from build123d import *

# Parameters (mm, degrees)
SKETCH1_W                       = 15.875
SKETCH1_H                       = 34.925
BASE_FLANGE1_DEPTH              = 3.03784
F_9_32_0_28125_DIAMETER_HOLE1_D = 7.14375
BREAK_CORNER1_DEPTH             = 3.03784


# Read off the part's stored shape, not the designer's step: Break-Corner1
# Sheet-metal steps are written as plain solids
with BuildPart() as part:
    # Sketch1 → Base-Flange1 (new body)
    with BuildSketch(Plane.XY):
        Rectangle(SKETCH1_W, SKETCH1_H)
    extrude(amount=BASE_FLANGE1_DEPTH)

    # 9/32 (0.28125) Diameter Hole1 (through all)
    with Locations(Plane.XY.offset(3.03784)):
        with Locations((0, 9.525), (0, -9.525)):
            Hole(F_9_32_0_28125_DIAMETER_HOLE1_D / 2)

    # Break-Corner1 outline → Break-Corner1 (cut)
    with BuildSketch(Plane.XY):
        with BuildLine():
            Line((-7.9375, -17.4625), (-3.175, -17.4625))
            ThreePointArc((-3.175, -17.4625), (-6.542596045, -16.067596045), (-7.9375, -12.7))
            Line((-7.9375, -12.7), (-7.9375, -17.4625))
        make_face()
        with BuildLine():
            ThreePointArc((7.9375, -12.7), (6.542596045, -16.067596045), (3.175, -17.4625))
            Line((3.175, -17.4625), (7.9375, -17.4625))
            Line((7.9375, -17.4625), (7.9375, -12.7))
        make_face()
        with BuildLine():
            Line((-7.9375, 17.4625), (-7.9375, 12.7))
            ThreePointArc((-7.9375, 12.7), (-6.542596045, 16.067596045), (-3.175, 17.4625))
            Line((-3.175, 17.4625), (-7.9375, 17.4625))
        make_face()
        with BuildLine():
            ThreePointArc((3.175, 17.4625), (6.542596045, 16.067596045), (7.9375, 12.7))
            Line((7.9375, 12.7), (7.9375, 17.4625))
            Line((7.9375, 17.4625), (3.175, 17.4625))
        make_face()
    extrude(amount=BREAK_CORNER1_DEPTH, mode=Mode.SUBTRACT)


solid = part.part
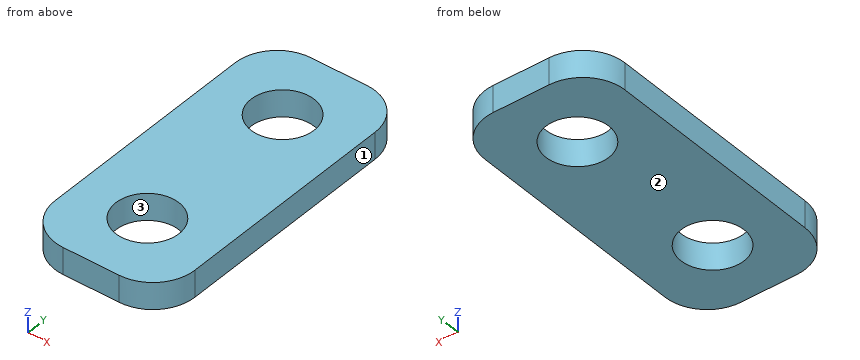
For this review, take the finished solid that the model builds, in its own axes (mm). Face numbers are marked on the shaded views. Give positions to 0.01 mm unless a question says otherwise; leave off trailing zeros. Loops run counter-clockwise (first coordinate to the right, second up) from the corner with the lowest first, then second, coordinate; pieces in that order, holes last. Notation, with made-up numbers: M 40,39 L 72,39 A12 cw 72,62 Z; hole C 17,-39 d6. An arc over 180 degrees is marked long. Put each result on its own line as item: value. Start each with the question number.
(1) Add section A-A, the plane x = 0. Write out the cut boundary in (y, z), then the cut area to 3 significant figures.
(2) Wall thickness on L1, parallel to Y at x = 0, z = 1.15; L2, parallel to Y at x = 3, z = 2; L3, parallel to X at y = -7, z = 2.35: over which ranges is each line inside the solid? List them lowest first.
(3) The part is to be moulded in two halves that separate along X. For the marked faces 1, 2 and 3, say which applies: +X half, -X half, draft (parallel to the pull), parting line (faces both ways), or undercut.
(4) For pin 1 (1 mm diameter, centred on x = -6, z = 2.5, fed in from -Y), flat-tipped, find the tip position at first contact; note if it passes through.
(5) Add section B-B, the plane z = 2.25. Write out the cut boundary in (x, y) (1 decimal), then the cut area to 3 significant figures.
(6) Add section C-C, the plane y = -8. Write out the cut boundary in (x, z).
(7) Add section D-D, the plane x = -1.75. Write out the cut boundary in (y, z).
Result:
1. outline: M -17.46,0 L -13.1,0 L -13.1,3.04 L -17.46,3.04 Z; M -5.95,0 L 5.95,0 L 5.95,3.04 L -5.95,3.04 Z; M 13.1,0 L 17.46,0 L 17.46,3.04 L 13.1,3.04 Z
1. area: 62.7 mm^2
2. L1: y = -17.46 to -13.1, -5.95 to 5.95, 13.1 to 17.46
2. L2: y = -17.46 to -11.46, -7.59 to 7.59, 11.46 to 17.46
2. L3: x = -7.94 to -2.53, 2.53 to 7.94
3. face 1: +X half
3. face 2: draft
3. face 3: undercut
4. pin 1: stops at y = -16.86
5. outline: M -7.9,-12.7 A4.8 ccw -3.2,-17.5 L 3.2,-17.5 A4.8 ccw 7.9,-12.7 L 7.9,12.7 A4.8 ccw 3.2,17.5 L -3.2,17.5 A4.8 ccw -7.9,12.7 Z; hole C 0,-9.5 d7.1; hole C 0,9.5 d7.1
5. area: 455 mm^2
6. outline: M -7.94,0 L -3.23,0 L -3.23,3.04 L -7.94,3.04 Z; M 3.23,0 L 7.94,0 L 7.94,3.04 L 3.23,3.04 Z
7. outline: M -17.46,0 L -12.64,0 L -12.64,3.04 L -17.46,3.04 Z; M -6.41,0 L 6.41,0 L 6.41,3.04 L -6.41,3.04 Z; M 12.64,0 L 17.46,0 L 17.46,3.04 L 12.64,3.04 Z
